Source: CAD feature listing. Evaluate the final solid. Frame: model axes, mm. Face numbers are marked on the shaded views. A direction names the side the tool comes from. Round coordinates to 2 decimals unless told otherwise and drop trailing zeros. Write each loop counter-clockwise with the first axis right and the second up, starting at its lowest first coordinate (ties: lowest second). Pieces come first, ordered by that corner, then holes. Notation, with made-up numbers: M 78.5,69 L 131.5,69 A36 ccw 131.5,105 Z; hole C -30.75,38.5 d9. An arc over 180 degrees is marked long. Answer in a Markdown table with one row per item. Add a question column.
Item 1: Material intervals for probe 1 along Y at (x, z) = (0, 14.75); probe 2 along Z at (x, y) = (-1.35, -1.9); probe 3 along X at (y, z) = (-0.7, 1.5), sorted ascending.
Item 2: Mould query, pull axis Z, two halves, no side actions, for the marked faces 3, 4 and 5. Classes: released by +Z, released by -Z, zero draft, split by the parting line, or undercut.
Item 3: Contact query for a flat-ended pin moving along its axis: pin 1 (2 mm diameter, centred on x = -0.5, y = 2.5, fed in from +Z). Output: stop coordinate, or through.
Item 4: Cut plane C-C on z = 8. Return loops of the section in (x, y), and give its area (3 significant figures).
Item 5: Set-up query: the marked faces 1 and 2. Return all of +Z, -Z, +X, -X, +Y, -Y with unobstructed straight access to the full face (end or side cutting, diameter ignored); none if empty.
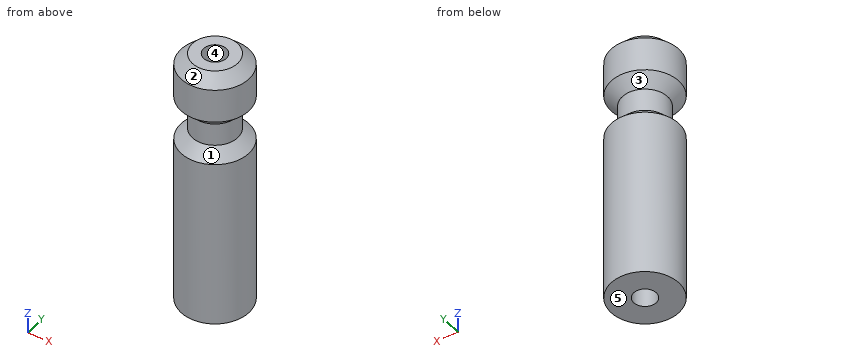
from build123d import *

# Parameters (mm, degrees)
F0_R     = 3
F1_DEPTH = 16
F2_R     = 2
F3_DEPTH = 2
F4_R     = 3
F5_DEPTH = 5
F6_SIZE  = 0.99999
F7_R     = 1
F8_DEPTH = 25


# Not quite as in the source:
# - a fillet or chamfer is up to 0.001 mm smaller than in the source, because OpenCascade refuses the exact size


with BuildPart() as f1:
    # F0 (on Top) → F1 (new body)
    with BuildSketch(Plane.XY):
        Circle(F0_R)
    extrude(amount=F1_DEPTH)

    # F2 (on face) → F3 (join)
    with BuildSketch(Plane.XY.offset(16)):
        Circle(F2_R)
    extrude(amount=F3_DEPTH)

    # F4 (on face) → F5 (join)
    with BuildSketch(Plane.XY.offset(18)):
        Circle(F4_R)
    extrude(amount=F5_DEPTH)

    # F6 (size 1 in the source; OpenCascade refuses exactly that, so slightly less here)
    f6_edges = [f1.edges().sort_by_distance(p)[0] for p in [
        (-3, 0, 23),
        (-3, 0, 18),
        (-3, 0, 16),
    ]]
    chamfer(f6_edges, length=F6_SIZE)

    # F7 (on face) → F8 (cut)
    with BuildSketch(Plane(origin=(0, 0, 0), x_dir=(1, 0, 0), z_dir=(0, 0, -1))):
        Circle(F7_R)
    extrude(amount=-F8_DEPTH, mode=Mode.SUBTRACT)


solid = f1.part
Results below:
| question | item | result |
|---|---|---|
| 1 | probe 1 | -3 to -1, 1 to 3 |
| 1 | probe 2 | 0 to 15.67, 18.33 to 22.67 |
| 1 | probe 3 | -2.92 to -0.71, 0.71 to 2.92 |
| 2 | face 3 | undercut |
| 2 | face 4 | zero draft |
| 2 | face 5 | released by -Z |
| 3 | pin 1 | z = 23 |
| 4 | outline | C 0,0 d6; hole C 0,0 d2 |
| 4 | area | 25.1 mm2 |
| 5 | face 1 | none |
| 5 | face 2 | +Z |
